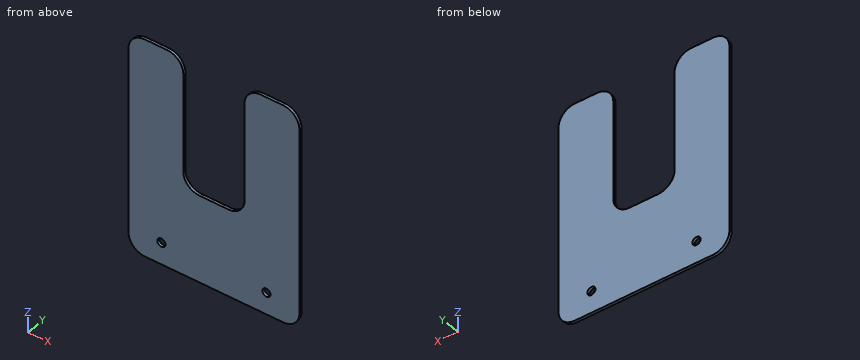
Autodesk Fusion 360 part; units mm, degrees
sketch "Sketch1" plane through (0, 0, 0) normal (0, 1, 0) x (1, 0, 0)
  line L0 (0, 0) -> (35.56, 0)
  line L1 (0, 0) -> (0, -76.2)
  line L2 (35.56, 0) -> (35.56, -76.2)
  line L3 (0, -76.2) -> (-31.75, -76.2)
  line L4 (35.56, -76.2) -> (67.31, -76.2)
  line L5 (-31.75, -76.2) -> (-31.75, 50.8)
  line L6 (67.31, -76.2) -> (67.31, 50.8)
  line L7 (-31.75, 50.8) -> (67.31, 50.8)
  line L8 (-31.75, 50.8) -> (-12.7, 50.8) construction
  line L9 (-12.7, 50.8) -> (-12.7, 38.1) construction
  line L10 (67.31, 50.8) -> (48.26, 50.8) construction
  line L11 (48.26, 50.8) -> (48.26, 38.1) construction
  circle A0 centre (48.26, 38.1) radius 2.3813
  circle A1 centre (-12.7, 38.1) radius 2.3813
  dimension "d2" = 76.2
  dimension "d3" = 76.2
  dimension "d4" = 31.75
  dimension "d5" = 31.75
  dimension "d6" = 127
  dimension "d7" = 127
  dimension "d8" = 19.05
  dimension "d9" = 4.7625
  dimension "d10" = 4.7625
extrude "Extrude1" add sketch "Sketch1" along normal blind 1.5875 makes body 1
fillet "Fillet1" radius 9.525 8 edges at (0, 0.7937, 0) (35.56, 0.7937, 0) (-31.75, 0.7937, 76.2) (0, 0.7937, 76.2) (35.56, 0.7937, 76.2) (67.31, 0.7937, 76.2) (67.31, 0.7937, -50.8) (-31.75, 0.7937, -50.8) on bodies 1
copy_body "Body->Comp1" bodies 1 removing the originals makes body 2 in component "Component"
component "Component" placed x (1, 0, 0) y (0, 1, 0) z (0, 0, 1) at (0, 0, 0)
equation "d11 = ( 1 / 16 ) * 1 in"
Geometry check sheet. Reference: the model listing, model coordinates, mm. Give positions to 0.01 mm unless a question says otherwise; leave off trailing zeros. Write each loop counter-clockwise with the first axis right and the second up, starting at its lowest first coordinate (ties: lowest second). Pieces come first, ordered by that corner, then holes.
1) Gauge pin test, flat ends, axial feed: pin 1 (4 mm diameter, centred on x = 48.26, z = -38.1, fed in from +Y); pin 2 (0.5 mm diameter, centred on x = 18, y = 1, fed in from +Z). Record the tip position at first contact, or that the pin passes through.
2) Section check D-D, the plane z = 57. Record the boundary of the cut face in (x, y).
3) Section check A-A, the plane x = 48.26. Record the boundary of the cut face in (y, z).
4) Material ranges on L1, parallel to X at y = 1.1, z = -38.1; L2, parallel to X at y = 0.65, z = 10; L3, parallel to Z at x = 48.26, y = 0.75, recorded low to high.
5) Section check B-B, the plane z = -38.1. Record the boundary of the cut face in (x, y), and give its area (3 significant figures).
6) Section check C-C, the plane y = 1.05. Record the boundary of the cut face in (x, z) (3 decimals).
Computed:
1. pin 1: passes through
1. pin 2: stops at z = 0
2. outline: (-31.75, 0) - (0, 0) - (0, 1.59) - (-31.75, 1.59) - close; (35.56, 0) - (67.31, 0) - (67.31, 1.59) - (35.56, 1.59) - close
3. outline: (0, -50.8) - (1.59, -50.8) - (1.59, -40.48) - (0, -40.48) - close; (0, -35.72) - (1.59, -35.72) - (1.59, 76.2) - (0, 76.2) - close
4. L1: x = -31.75 to -15.08, -10.32 to 45.88, 50.64 to 67.31
4. L2: x = -31.75 to 0, 35.56 to 67.31
4. L3: z = -50.8 to -40.48, -35.72 to 76.2
5. outline: (-31.75, 0) - (-15.08, 0) - (-15.08, 1.59) - (-31.75, 1.59) - close; (-10.32, 0) - (45.88, 0) - (45.88, 1.59) - (-10.32, 1.59) - close; (50.64, 0) - (67.31, 0) - (67.31, 1.59) - (50.64, 1.59) - close
5. area: 142 mm2
6. outline: (-31.75, -41.275) arc R9.525 ccw to (-22.225, -50.8) - (57.785, -50.8) arc R9.525 ccw to (67.31, -41.275) - (67.31, 66.675) arc R9.525 ccw to (57.785, 76.2) - (45.085, 76.2) arc R9.525 ccw to (35.56, 66.675) - (35.56, 9.525) arc R9.525 cw to (26.035, 0) - (9.525, 0) arc R9.525 cw to (0, 9.525) - (0, 66.675) arc R9.525 ccw to (-9.525, 76.2) - (-22.225, 76.2) arc R9.525 ccw to (-31.75, 66.675) - close; hole circle Ø4.763 at (-12.7, -38.1); hole circle Ø4.763 at (48.26, -38.1)
